Source: CAD feature listing. Evaluate the final solid. Frame: model axes, mm. Face numbers are marked on the shaded views. A direction names the side the tool comes from. Give positions to 0.01 mm unless a question says otherwise; leave off trailing zeros. Write each loop counter-clockwise with the first axis right and the second up, starting at its lowest first coordinate (ties: lowest second). Pieces come first, ordered by that corner, then holes. Notation, with made-up numbers: (50, 0) - (79, 0) arc R18 ccw to (79, 10) - close; hole circle Ø10 at (89.5, 19). An arc over 180 degrees is marked (long way). One line per question, with ' | ' between items. Start each with the question number.
(1) Section C-C, the plane y = 5. Return loops of the section in (x, z).
(2) Section A-A, the plane y = 36. Return loops of the section in (x, z).
(3) Section D-D, the plane x = 2.5. Return loops of the section in (y, z).
(4) Access query for the marked faces 4, 5, 6 and 7. Directions: +Z, -Z, +X, -X, +Y, -Y. A direction counts if a zero-diameter tool reaches every point of the face in a straight line with its end or side. Return the directions, or none.
(5) Ray query, line 1 (X direction, y = 40, z = 74.5); line 2 (Y direction, x = -6.5, z = 65); line 3 (X direction, y = 1, z = 38). Return the intervals inside material, ascending. Write a range as [from, to].
(6) Draft query along X for the marked faces 1, 2 and 3. Return one class per face: +X half, -X half, draft (parallel to the pull), parting line (faces both ways), or undercut.
(7) Pin query (flat end, axial travel): pin 1 (5 mm diameter, centred on x = 0, z = 34, fed in from -Y); pin 2 (8 mm diameter, centred on y = 20, z = 60.5, fed in from +X); pin 3 (6 mm diameter, centred on y = 21.7, z = 15, fed in from -X); pin 4 (10 mm diameter, centred on x = -5.5, y = 35.5, fed in from -Z). Return the tip coordinate at first contact, or that it passes through.
(8) Section B-B, the plane z = 65. State how many separate pieces and enclosed holes the cut face has, plus the area to 3 significant figures.
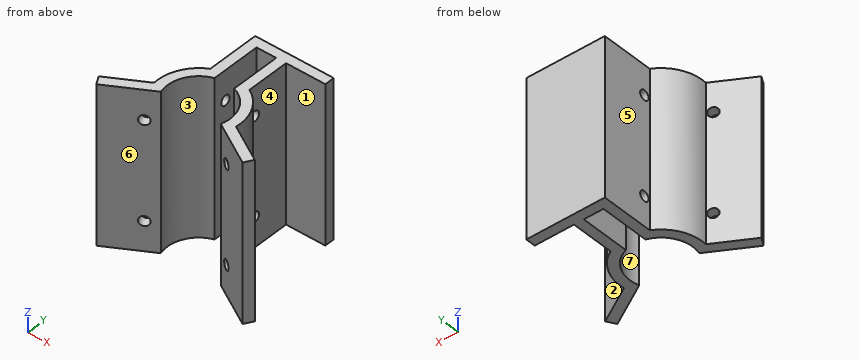
```python
from build123d import *

# Parameters (mm, degrees)
BOSS_EXTRUDE1_DEPTH            = 80
F_5_0MM_DOWEL_HOLE1_AT_2_COUNT = 2
F_5_0MM_DOWEL_HOLE1_AT_2_PITCH = 50
SKETCH5_W                      = 2.5
SKETCH5_H                      = 34.757041555
F_5_0MM_DOWEL_HOLE2_AT_2_COUNT = 2
F_5_0MM_DOWEL_HOLE2_AT_2_PITCH = 50
MIRROR2_COPY_1_SKETCH_W        = 2.5
MIRROR2_COPY_1_SKETCH_H        = 34.757041555


with BuildPart() as part:
    # Sketch1 → Boss-Extrude1 (new body)
    with BuildSketch(Plane.XY):
        with BuildLine():
            Line((-5, 15.198684154), (-5, 40.198684154))
            Line((-5, 40.198684154), (5, 40.198684154))
            Line((5, 40.198684154), (5, 15.198684154))
            ThreePointArc((5, 15.198684154), (14.229023395, 7.316754283), (15.270817283, -4.775158585))
            Line((15.270817283, -4.775158585), (37.257041555, -17.468911087))
            Line((37.257041555, -17.468911087), (39.757041555, -13.138784068))
            Line((39.757041555, -13.138784068), (20.88016837, -2.240216253))
            ThreePointArc((20.88016837, -2.240216253), (18.589915709, 9.768061933), (10, 18.466185313))
            Line((10, 18.466185313), (10, 40.198684154))
            Line((10, 40.198684154), (30, 40.198684154))
            Line((30, 40.198684154), (30, 45.198684154))
            Line((30, 45.198684154), (-10, 45.198684154))
            Line((-10, 45.198684154), (-10, 18.466185313))
            ThreePointArc((-10, 18.466185313), (-18.589915709, 9.768061933), (-20.88016837, -2.240216253))
            Line((-20.88016837, -2.240216253), (-39.757041555, -13.138784068))
            Line((-39.757041555, -13.138784068), (-37.257041555, -17.468911087))
            Line((-37.257041555, -17.468911087), (-15.270817283, -4.775158585))
            ThreePointArc((-15.270817283, -4.775158585), (-14.229023395, 7.316754283), (-5, 15.198684154))
        make_face()
    extrude(amount=BOSS_EXTRUDE1_DEPTH)

    # Sketch3 → Ø5.0mm Dowel Hole1 (revolve, cut)
    with BuildSketch(Plane(origin=(20.899982408, -8.025158585, 65), x_dir=(0.866025403784438, -0.5000000000000012, 0), z_dir=(0, 0, 1))):
        Polygon((0, 0), (0, 11.502151548), (2.5, 10), (2.5, 0), align=None)
    f_5_0mm_dowel_hole1 = revolve(axis=Axis((17.724982408, -13.524419899, 65), (0.5000000000000012, 0.8660254037844379, 0)), mode=Mode.SUBTRACT)

    # Ø5.0mm Dowel Hole1 at 2: Ø5.0mm Dowel Hole1 ×2
    with Locations(*[(0, 0, -i * F_5_0MM_DOWEL_HOLE1_AT_2_PITCH) for i in range(1, F_5_0MM_DOWEL_HOLE1_AT_2_COUNT)]):
        add(f_5_0mm_dowel_hole1, mode=Mode.SUBTRACT)

    # Mirror1: Ø5.0mm Dowel Hole1 across plane
    add(f_5_0mm_dowel_hole1.mirror(Plane(origin=(0, 0, 0), x_dir=(0, 0, 1), z_dir=(1, 0, 0))), mode=Mode.SUBTRACT)

    # Mirror1 copy 1 sketch → Mirror1 copy 1 (revolve, cut)
    with BuildSketch(Plane(origin=(-20.899982408, -8.025158585, 15), x_dir=(-0.866025403784438, -0.5000000000000012, 0), z_dir=(0, 0, 1))):
        Polygon((0, 0), (0, -11.502151548), (2.5, -10), (2.5, 0), align=None)
    revolve(axis=Axis((-17.724982408, -13.524419899, 15), (0.5000000000000012, -0.8660254037844379, 0)), mode=Mode.SUBTRACT)

    # Sketch5 → Ø5.0mm Dowel Hole2 (revolve, cut)
    with BuildSketch(Plane(origin=(-5, 21.698684154, 15), x_dir=(0, 0, -1), z_dir=(0, 1, 0))):
        with Locations((1.25, 17.378520778)):
            Rectangle(SKETCH5_W, SKETCH5_H)
    f_5_0mm_dowel_hole2 = revolve(axis=Axis((1.35, 21.698684154, 15), (-1, 0, 0)), mode=Mode.SUBTRACT)

    # Ø5.0mm Dowel Hole2 at 2: Ø5.0mm Dowel Hole2 ×2
    with Locations(*[(0, 0, i * F_5_0MM_DOWEL_HOLE2_AT_2_PITCH) for i in range(1, F_5_0MM_DOWEL_HOLE2_AT_2_COUNT)]):
        add(f_5_0mm_dowel_hole2, mode=Mode.SUBTRACT)

    # Mirror2: Ø5.0mm Dowel Hole2 across plane
    add(f_5_0mm_dowel_hole2.mirror(Plane(origin=(0, 0, 0), x_dir=(0, 0, 1), z_dir=(1, 0, 0))), mode=Mode.SUBTRACT)

    # Mirror2 copy 1 sketch → Mirror2 copy 1 (revolve, cut)
    with BuildSketch(Plane(origin=(5, 21.698684154, 65), x_dir=(0, 0, -1), z_dir=(0, 1, 0))):
        with Locations((1.25, -17.378520778)):
            Rectangle(MIRROR2_COPY_1_SKETCH_W, MIRROR2_COPY_1_SKETCH_H)
    revolve(axis=Axis((-1.35, 21.698684154, 65), (-1, 0, 0)), mode=Mode.SUBTRACT)


solid = part.part
```
Check sheet entries:
1) outline: (-20.4, 0) - (-15.2, 0) - (-15.2, 80) - (-20.4, 80) - close; (15.2, 0) - (20.4, 0) - (20.4, 80) - (15.2, 80) - close
2) outline: (-10, 0) - (-5, 0) - (-5, 80) - (-10, 80) - close; (5, 0) - (10, 0) - (10, 80) - (5, 80) - close
3) outline: (40.2, 0) - (45.2, 0) - (45.2, 80) - (40.2, 80) - close
4) face 4: +Z, -Z, +X | face 5: +Z, -Z, -X, +Y | face 6: +Z, -Z, -Y | face 7: +Z, -Z
5) line 1: [-10, -5], [5, 10] | line 2: [14.62, 19.2], [24.2, 45.2] | line 3: [-20.98, -15.97], [15.97, 20.98]
6) face 1: draft | face 2: +X half | face 3: undercut
7) pin 1: y = 40.2 | pin 2: x = 13.6 | pin 3: x = -10 | pin 4: z = 0
8) separate pieces: 5 | enclosed holes: 0 | area: 817 mm²
